from build123d import *

# Parameters (mm, degrees)
BOSS_EXTRUDE1_DEPTH = 30
SKETCH3_R           = 1.5
SKETCH3_W           = 6.2
SKETCH3_H           = 10
MAKERBEAMFIX_DEPTH  = 6.5
SKETCH4_R           = 1.25
FIXHOLES_DEPTH      = 6.5
SKETCH5_W           = 5
SKETCH5_H           = 16
PINFIXHOLES_DEPTH   = 1.5
LPATTERN1_COUNT     = 2
LPATTERN1_PITCH     = 25


with BuildPart() as part:
    # Sketch1 → Boss-Extrude1 (new body, symmetric)
    with BuildSketch(Plane.XY):
        Polygon((-11.2, 1), (-1.45, 1), (-1.45, 0), (1.45, 0), (1.45, 1), (11.2, 1), (11.2, 5.5), (-11.2, 5.5), align=None)
    extrude(amount=BOSS_EXTRUDE1_DEPTH, both=True)

    # Sketch3 → MakerBeamFix (cut, through all)
    with BuildSketch(Plane(origin=(0, 5.5, 0), x_dir=(1, 0, 0), z_dir=(0, 1, 0))):
        with Locations((0, 25)):
            Circle(SKETCH3_R)
        with Locations((-8.1, 25)):
            Rectangle(SKETCH3_W, SKETCH3_H)
        with Locations((8.1, 25)):
            Rectangle(SKETCH3_W, SKETCH3_H)
    extrude(amount=-MAKERBEAMFIX_DEPTH, mode=Mode.SUBTRACT)

    # Sketch4 → FixHoles (cut, through all)
    with BuildSketch(Plane(origin=(0, 5.5, 0), x_dir=(1, 0, 0), z_dir=(0, 1, 0))):
        with Locations((-8.6, 17.5)):
            Circle(SKETCH4_R)
        with Locations((8.6, 17.5)):
            Circle(SKETCH4_R)
        with Locations((-8.6, -2.7)):
            Circle(SKETCH4_R)
        with Locations((8.6, -2.7)):
            Circle(SKETCH4_R)
    fixholes = extrude(amount=-FIXHOLES_DEPTH, mode=Mode.SUBTRACT)

    # Sketch5 → PinFixHoles (cut)
    with BuildSketch(Plane(origin=(0, 5.5, 0), x_dir=(1, 0, 0), z_dir=(0, 1, 0))):
        with Locations((-8.7, 7.5)):
            Rectangle(SKETCH5_W, SKETCH5_H)
        with Locations((8.7, 7.5)):
            Rectangle(SKETCH5_W, SKETCH5_H)
    pinfixholes = extrude(amount=-PINFIXHOLES_DEPTH, mode=Mode.SUBTRACT)

    # LPattern1: FixHoles, PinFixHoles ×2
    with Locations(*[(0, 0, i * LPATTERN1_PITCH) for i in range(1, LPATTERN1_COUNT)]):
        add(fixholes, mode=Mode.SUBTRACT)
        add(pinfixholes, mode=Mode.SUBTRACT)


solid = part.part
Input: part model. Units: mm. Frame: model coordinates. A direction names the side the tool comes from. Coordinates: 2 decimals unless noted, no trailing zeros. Loops run counter-clockwise (first coordinate to the right, second up) from the corner with the lowest first, then second, coordinate; pieces in that order, holes last.
(1) Section C-C on y = 1.7. Count the separate pieces of the cut face and the enclosed holes in it, then the cut area to 3 significant figures.
(2) Set-up query: faces 5 (the face through (8, 3, -20)), 6 (the face through (-9, 4, 17)), 7 (the face through (-1.45, 0.5, -27.7)), 8 (the face through (1.45, 0.5, -27.7)). Return all of +Z, -Z, +X, -X, +Y, -Y with unobstructed straight access to the full face (end or side cutting, diameter ignored); none if empty.
(3) Section A-A on z = -17.5. Return the cut outline in (x, y).
(4) Material intervals for probe 1 along X at (y, z) = (4.55, -17.5); probe 2 along Z at (x, y) = (8.6, 2.3); probe 3 along X at (y, z) = (3.55, -25), sorted ascending.
(5) Section B-B on x = 0. Return the cut outline in (y, z).
(6) Pull-direction query (X, two-part tool) for faces 1 (the face through (8.33, 3.28, -16.28)), 2 (the face through (6.2, 5, 18)), 3 (the face through (-9, 5, -15.5)), 4 (the face through (1.43, 2.79, -25.45)); classes: released by +X, released by -X, zero draft, split by the parting line, or undercut.
(7) Section D-D on x = -8.6. Return the cut outline in (y, z), then the cut area to 3 significant figures.
(8) First-contact query: pin 1 Ø1.5 at (x, y) = (8, 3.5) entering from -Z; pin 2 Ø3 at (x, z) = (-8.6, 27.7) entering from -Y; pin 3 Ø1.3 at (y, z) = (3, -23.5) entering from +X. Flat tips, straight axial feed; report the tip coordinate or a pass-through.
Data:
1. separate pieces: 1
1. enclosed holes: 9
1. area: 1,170 mm2
2. face 5: -Z, +X, +Y, -Y
2. face 6: -X, +Y
2. face 7: +Z, -Z, -X, -Y
2. face 8: +Z, -Z, +X, -Y
3. outline: (-11.2, 1) - (-9.85, 1) - (-9.85, 5.5) - (-11.2, 5.5) - close; (-7.35, 1) - (-1.45, 1) - (-1.45, 0) - (1.45, 0) - (1.45, 1) - (7.35, 1) - (7.35, 5.5) - (-7.35, 5.5) - close; (9.85, 1) - (11.2, 1) - (11.2, 5.5) - (9.85, 5.5) - close
4. probe 1: x = -11.2 to -9.85, -7.35 to 7.35, 9.85 to 11.2
4. probe 2: z = -20 to -18.75, -16.25 to 1.45, 3.95 to 6.25, 8.75 to 26.45, 28.95 to 30
4. probe 3: x = -5 to -1.5, 1.5 to 5
5. outline: (0, -30) - (5.5, -30) - (5.5, -26.5) - (0, -26.5) - close; (0, -23.5) - (5.5, -23.5) - (5.5, 30) - (0, 30) - close
6. face 1: undercut
6. face 2: released by +X
6. face 3: zero draft
6. face 4: undercut
7. outline: (1, -20) - (5.5, -20) - (5.5, -18.75) - (1, -18.75) - close; (1, -16.25) - (5.5, -16.25) - (5.5, -15.5) - (4, -15.5) - (4, 0.5) - (5.5, 0.5) - (5.5, 1.45) - (1, 1.45) - close; (1, 3.95) - (5.5, 3.95) - (5.5, 6.25) - (1, 6.25) - close; (1, 8.75) - (5.5, 8.75) - (5.5, 9.5) - (4, 9.5) - (4, 25.5) - (5.5, 25.5) - (5.5, 26.45) - (1, 26.45) - close; (1, 28.95) - (5.5, 28.95) - (5.5, 30) - (1, 30) - close
7. area: 132 mm2
8. pin 1: stops at z = -20
8. pin 2: stops at y = 1
8. pin 3: stops at x = 5
